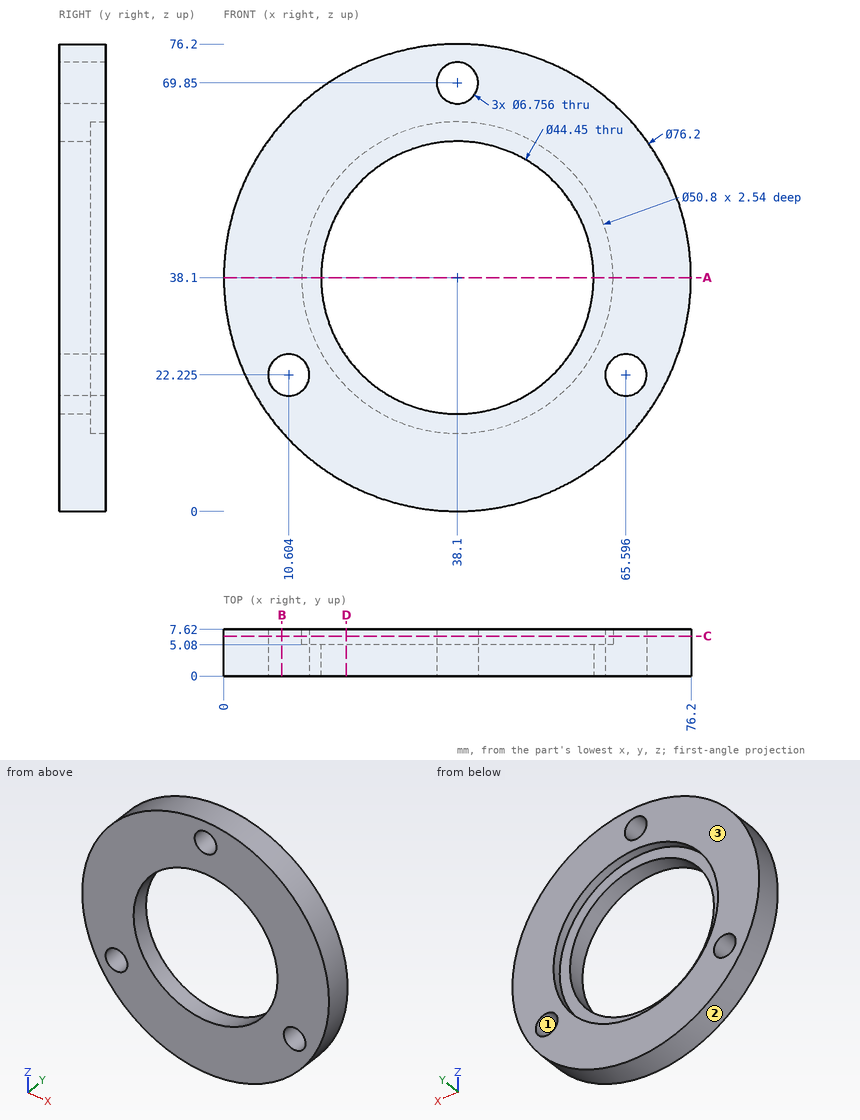
Could you check a few things on this drawing? It's one solid part, dimensions in mm from its lowest x, y, z. Coordinates: 2 decimals unless noted, no trailing zeros. Loops run counter-clockwise (first coordinate to the right, second up) from the corner with the lowest first, then second, coordinate; pieces in that order, holes last. Notation, with made-up numbers: (48.25, -5.5) - (54.25, -5.5) arc R25 ccw to (54.25, 18.5) - close; hole circle Ø3 at (-34, 43). An arc over 180 degrees is marked (long way). Answer as a JSON object with one key per item and string values. Group by question number.
Item 1: For pin 1 (3 mm diameter, centred on y = 1, z = 24.5, fed in from +X); pin 2 (3 mm diameter, centred on y = 3.5, z = 55, fed in from -X); pin 3 (5.5 mm diameter, centred on x = 10.6, z = 22.22, fed in from -Y); pin 4 (2 mm diameter, centred on y = 3.5, z = 30.5, fed in from -X), each with a flat end and sliding along its axis, tell me the tip position at first contact or that it passes through.
Item 2: If we mould it in two halves opening along X, with no side actions, what happens to the marked faces 1, 2 and 3? For each: released by +X, released by -X, zero draft, split by the parting line, or undercut.
Item 3: If I drill on L1, parallel to Z at x = 38.1, y = 5.8; L2, parallel to Z at x = 39, y = 4.25 (1 decimal); L3, parallel to X at y = 1.5, z = 26.5, over which ranges is the centre line in solid material (lowest first)? Write a range as from..to.
Item 4: If we section it at B-B (x = 9.5): List the corners of the cut face in (y, z) for me.
Item 5: If we section it at A-A (z = 38.1): List the corners of the cut face in (x, y) for me (1 decimal), plus the area to 3 significant figures.
Item 6: If we section it at D-D (x = 20): List the corners of the cut face in (y, z) for me.
Item 7: If we section it at C-C (y = 6.5): State how many separate pieces and enclosed holes the cut face has, plus the area to 3 significant figures.
Returned:
{
 "1": {"pin 1": "stops at x = 74.23", "pin 2": "stops at x = 3.25", "pin 3": "passes through", "pin 4": "stops at x = 0.58"},
 "2": {"face 1": "undercut", "face 2": "split by the parting line", "face 3": "zero draft"},
 "3": {"L1": "z = 0..12.7, 63.5..66.47, 73.23..76.2", "L2": "z = 0..15.9, 60.3..66.6, 73.1..76.2", "L3": "x = 1.81..19.14, 57.06..74.39"},
 "4": {"outline": "(0, 12.93) - (7.62, 12.93) - (7.62, 19.03) - (0, 19.03) - close; (0, 25.42) - (7.62, 25.42) - (7.62, 63.27) - (0, 63.27) - close"},
 "5": {"outline": "(0, 0) - (15.9, 0) - (15.9, 5.1) - (12.7, 5.1) - (12.7, 7.6) - (0, 7.6) - close; (60.3, 0) - (76.2, 0) - (76.2, 7.6) - (63.5, 7.6) - (63.5, 5.1) - (60.3, 5.1) - close", "area": "226 mm²"},
 "6": {"outline": "(0, 4.57) - (7.62, 4.57) - (7.62, 20.28) - (5.08, 20.28) - (5.08, 25.2) - (0, 25.2) - close; (0, 51) - (5.08, 51) - (5.08, 55.92) - (7.62, 55.92) - (7.62, 71.63) - (0, 71.63) - close"},
 "7": {"separate pieces": "1", "enclosed holes": "4", "area": "2,430 mm²"}
}
